Input: part model. Units: mm. Frame: model coordinates. A direction names the side the tool comes from. Give positions to 0.01 mm unless a question says otherwise; leave off trailing zeros. Write each loop counter-clockwise with the first axis right and the second up, starting at its lowest first coordinate (ties: lowest second). Pieces come first, ordered by that corner, then holes. Notation, with made-up numbers: (20, 11) - (35, 11) arc R8 ccw to (35, 18) - close; hole circle Ø2 at (32, -9). An arc over 180 degrees is marked (long way). Use a Markdown table: item, result. Add a question column.
1. Mould query, pull axis Y, two halves, no side actions, for faces 1 (the cylindrical face through (-4.9, -1.5, 2.5)), 2 (the flat face through (-23, 77.5, 2)), 3 (the cylindrical face through (-11.834, 68.222, 2.465)). Classes: released by +Y, released by -Y, zero draft, split by the parting line, or undercut.
2. Section query A-A, the plane y = 12.5. Return loops of the section in (x, z).
3. Section query B-B, the plane y = 31. Return loops of the section in (x, z), plus the area to 4 significant figures.
4. Set-up query: faces 4 (the flat face through (-14, 0, 2)), 5 (the flat face through (-12.25, 25, 2)), 6 (the flat face through (-64, 0, 2)). Return all of +Z, -Z, +X, -X, +Y, -Y with unobstructed straight access to the full face (end or side cutting, diameter ignored); none if empty.
5. Pin query (flat end, axial travel): pin 1 (2 mm diameter, centred on y = 12, z = 4, fed in from +X); pin 2 (3 mm diameter, centred on y = 47, z = 1.5, fed in from +X); pin 3 (1.5 mm diameter, centred on x = -11, z = 2, fed in from -Y). Return the tip coordinate at first contact, or that it passes through.
6. Section query C-C, the plane z = 2.45. Count the separate pieces of the cut face and the enclosed holes in it, plus the area to 3 significant figures.
7. Material intervals for probe 1 along Y at (x, z) = (-5, 2.6); probe 2 along X at (y, z) = (12.5, 3.6); probe 3 along X at (y, z) = (21, 2.65), sorted ascending.
8. Section query D-D, the plane x = -25.5. Return loops of the section in (y, z), plus the area to 3 significant figures.
```python
from build123d import *

# Parameters (mm, degrees)
SKETCH1_R           = 2.1
SKETCH1_W           = 25
SKETCH1_H           = 5.1
BOSS_EXTRUDE1_DEPTH = 5
CUT_EXTRUDE2_DEPTH  = 5
SKETCH4_R           = 2.1
SKETCH4_R_2         = 4
BOSS_EXTRUDE2_DEPTH = 5
SKETCH5_W           = 25.4
SKETCH5_H           = 5
SKETCH5_H_2         = 5.4
CUT_EXTRUDE3_DEPTH  = 10


with BuildPart() as part:
    # Sketch1 → Boss-Extrude1 (new body)
    with BuildSketch(Plane.XY):
        with BuildLine():
            Line((-65, 61.5), (0, 61.5))
            Line((0, 61.5), (0, 0))
            Line((0, 0), (-1.877501001, 0))
            ThreePointArc((-1.877501001, 0), (-5, -1.5), (-8.122498999, 0))
            Line((-8.122498999, 0), (-20, 0))
            Line((-20, 0), (-20, 5))
            Line((-20, 5), (-45, 5))
            Line((-45, 5), (-45, 0))
            Line((-45, 0), (-56.877501001, 0))
            ThreePointArc((-56.877501001, 0), (-60, -1.5), (-63.122498999, 0))
            Line((-63.122498999, 0), (-65, 0))
            Line((-65, 0), (-65, 61.5))
        make_face()
        with Locations((-60, 56.5)):
            Circle(SKETCH1_R, mode=Mode.SUBTRACT)
        with Locations((-5, 56.5)):
            Circle(SKETCH1_R, mode=Mode.SUBTRACT)
        with Locations((-60, 46.5)):
            Circle(SKETCH1_R, mode=Mode.SUBTRACT)
        with Locations((-5, 46.5)):
            Circle(SKETCH1_R, mode=Mode.SUBTRACT)
        with Locations(Location((-5, 12.5, 0), (0, 0, 180))):
            Circle(SKETCH1_R, mode=Mode.SUBTRACT)
        with Locations(Location((-5, 2.5, 0), (0, 0, 180))):
            Circle(SKETCH1_R, mode=Mode.SUBTRACT)
        with Locations(Location((-60, 2.5, 0), (0, 0, 180))):
            Circle(SKETCH1_R, mode=Mode.SUBTRACT)
        with Locations(Location((-60, 12.5, 0), (0, 0, 180))):
            Circle(SKETCH1_R, mode=Mode.SUBTRACT)
        with Locations((-32.5, 12.5)):
            Rectangle(SKETCH1_W, SKETCH1_H, mode=Mode.SUBTRACT)
    extrude(amount=BOSS_EXTRUDE1_DEPTH)

    # Sketch3 → Cut-Extrude2 (cut)
    with BuildSketch(Plane(origin=(0, 0, 0), x_dir=(-1, 0, 0), z_dir=(0, 0, -1))):
        with BuildLine():
            Line((39.75, 15.05), (39.75, 34.55))
            ThreePointArc((39.75, 34.55), (26, 48.3), (12.25, 34.55))
            Line((12.25, 34.55), (12.25, 15.05))
            Line((12.25, 15.05), (39.75, 15.05))
        make_face()
    extrude(amount=-CUT_EXTRUDE2_DEPTH, mode=Mode.SUBTRACT)

    # Sketch4 → Boss-Extrude2 (add)
    with BuildSketch(Plane(origin=(0, 0, 0), x_dir=(-1, 0, 0), z_dir=(0, 0, -1))):
        Polygon((0, 41.5), (-17.5, 63.5), (-17.5, 77.5), (65, 77.5), (65, 61.5), (0, 61.5), align=None)
        with Locations((-11.5, 69.5)):
            Circle(SKETCH4_R, mode=Mode.SUBTRACT)
        with Locations((13.5, 69.5)):
            Circle(SKETCH4_R, mode=Mode.SUBTRACT)
        with Locations((26, 69.5)):
            Circle(SKETCH4_R_2, mode=Mode.SUBTRACT)
        with Locations((38.5, 69.5)):
            Circle(SKETCH4_R, mode=Mode.SUBTRACT)
    extrude(amount=-BOSS_EXTRUDE2_DEPTH)

    # Sketch5 → Cut-Extrude3 (cut)
    with BuildSketch(Plane(origin=(0, 0, 0), x_dir=(-1, 0, 0), z_dir=(0, 0, -1))):
        with Locations((32.5, 2.5)):
            Rectangle(SKETCH5_W, SKETCH5_H)
        with Locations((32.5, 12.55)):
            Rectangle(SKETCH5_W, SKETCH5_H_2)
    extrude(amount=-CUT_EXTRUDE3_DEPTH, mode=Mode.SUBTRACT)


solid = part.part
```
Result sheet:
| question | item | result |
|---|---|---|
| 1 | face 1 | released by -Y |
| 1 | face 2 | released by +Y |
| 1 | face 3 | undercut |
| 2 | outline | (-65, 0) - (-62.1, 0) - (-62.1, 5) - (-65, 5) - close; (-57.9, 0) - (-45.2, 0) - (-45.2, 5) - (-57.9, 5) - close; (-19.8, 0) - (-7.1, 0) - (-7.1, 5) - (-19.8, 5) - close; (-2.9, 0) - (0, 0) - (0, 5) - (-2.9, 5) - close |
| 3 | outline | (-65, 0) - (-39.75, 0) - (-39.75, 5) - (-65, 5) - close; (-12.25, 0) - (0, 0) - (0, 5) - (-12.25, 5) - close |
| 3 | area | 187.5 mm² |
| 4 | face 4 | +Z, -Z, -Y |
| 4 | face 5 | +Z, -Z |
| 4 | face 6 | +Z, -Z, -X, -Y |
| 5 | pin 1 | stops at x = 0 |
| 5 | pin 2 | stops at x = 5.57 |
| 5 | pin 3 | stops at y = 0 |
| 6 | separate pieces | 1 |
| 6 | enclosed holes | 13 |
| 6 | area | 4,190 mm² |
| 7 | probe 1 | y = -1.5 to 0.4, 4.6 to 10.4, 14.6 to 44.4, 48.6 to 54.4, 58.6 to 77.5 |
| 7 | probe 2 | x = -65 to -62.1, -57.9 to -45.2, -19.8 to -7.1, -2.9 to 0 |
| 7 | probe 3 | x = -65 to -39.75, -12.25 to 0 |
| 8 | outline | (5, 0) - (9.85, 0) - (9.85, 5) - (5, 5) - close; (48.29, 0) - (65.53, 0) - (65.53, 5) - (48.29, 5) - close; (73.47, 0) - (77.5, 0) - (77.5, 5) - (73.47, 5) - close |
| 8 | area | 131 mm² |
